Job drawing, mm, ordinate dimensions from the low corner. One solid piece. A direction names the side the tool comes from. Round coordinates to 2 decimals unless told otherwise and drop trailing zeros. Order: outer loops, then holes, each group sorted by start corner. A loop starts at its lowest first (then second) coordinate and runs counter-clockwise, first axis right, second up. Notation, with made-up numbers: (-17, -31) -> (-11, -31) arc R21 ccw to (-11, -11) -> close; hole circle Ø11 at (-15.5, 78). An arc over 180 degrees is marked (long way). Return JSON: item names as keys, results as strings. Group by question number.
Q1. Probe line 1 along X through (y, z) = (76, 28); line 2 along Y through (x, z) = (10, 38); line 3 along X through (y, z) = (103, 28). List the from-to ranges inside material, lowest first.
Q2. Mould opens along Y. For the marked faces 1, 2, 3 and 4 say: +Y half, -Y half, draft (parallel to the pull), parting line (faces both ways), or undercut.
Q3. Cut at D-D (x = 27). Write the cut outline in (y, z), then the cut area to 3 significant figures.
Q4. Cut at A-A (x = 63.5). Write the cut outline in (y, z) (3 decimals), then the cut area to 3 significant figures.
Q5. Flat gauge pins, fed straight in: pin 1 (3 mm diameter, centred on x = 18.5, z = 22, fed in from +Y); pin 2 (3 mm diameter, centred on y = 4, z = 15, fed in from -X); pin 3 (10 mm diameter, centred on y = 93, z = 15, fed in from -X); pin 4 (1.5 mm diameter, centred on x = 33.5, z = 11, fed in from +Y). Where does each tip first touch, or does it go through?
Q6. Cut at B-B (y = 76.2). Write the cut outline in (x, z).
Q7. Which spindle directions (+Z, -Z, +X, -X, +Y, -Y) get a long thin tool onto all of the face, cutting with end or side? Do the marked faces 5, 6 and 7. Say none if no direction does.
Q8. Cut at C-C (z = 19). Write the cut outline in (x, y) (3 decimals).
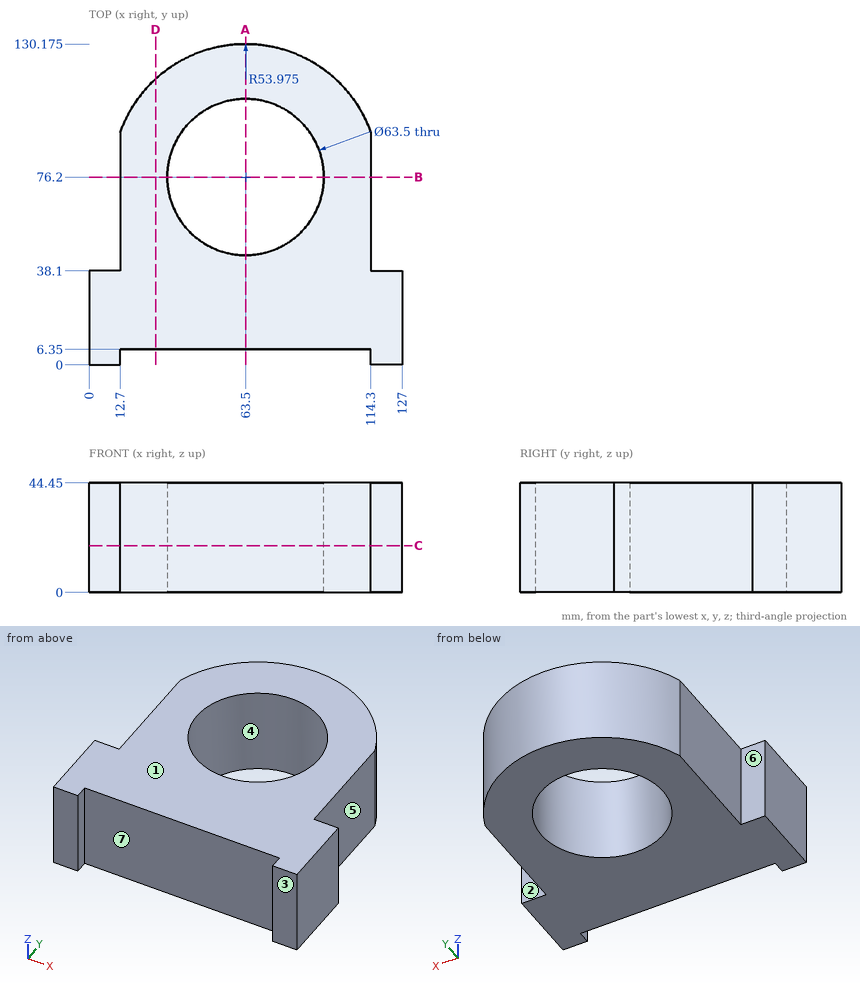
Solution:
{
 "1": {"line 1": "x = 12.7 to 31.75, 95.25 to 114.3", "line 2": "y = 0 to 38.1", "line 3": "x = 16.65 to 46.48, 80.52 to 110.35"},
 "2": {"face 1": "draft", "face 2": "+Y half", "face 3": "-Y half", "face 4": "undercut"},
 "3": {"outline": "(6.35, 0) -> (115.96, 0) -> (115.96, 44.45) -> (6.35, 44.45) -> close", "area": "4,870 mm²"},
 "4": {"outline": "(6.35, 0) -> (44.45, 0) -> (44.45, 44.45) -> (6.35, 44.45) -> close; (107.95, 0) -> (130.175, 0) -> (130.175, 44.45) -> (107.95, 44.45) -> close", "area": "2,680 mm²"},
 "5": {"pin 1": "stops at y = 108.15", "pin 2": "stops at x = 0", "pin 3": "stops at x = 12.7", "pin 4": "stops at y = 121.56"},
 "6": {"outline": "(12.7, 0) -> (31.75, 0) -> (31.75, 44.45) -> (12.7, 44.45) -> close; (95.25, 0) -> (114.3, 0) -> (114.3, 44.45) -> (95.25, 44.45) -> close"},
 "7": {"face 5": "+Z, -Z, +X, +Y", "face 6": "+Z, -Z, -X, +Y", "face 7": "+Z, -Z, -Y"},
 "8": {"outline": "(0, 0) -> (12.7, 0) -> (12.7, 6.35) -> (114.3, 6.35) -> (114.3, 0) -> (127, 0) -> (127, 38.1) -> (114.3, 38.1) -> (114.3, 94.439) arc R53.975 ccw to (12.7, 94.439) -> (12.7, 38.1) -> (0, 38.1) -> close; hole circle Ø63.5 at (63.5, 76.2)"}
}
